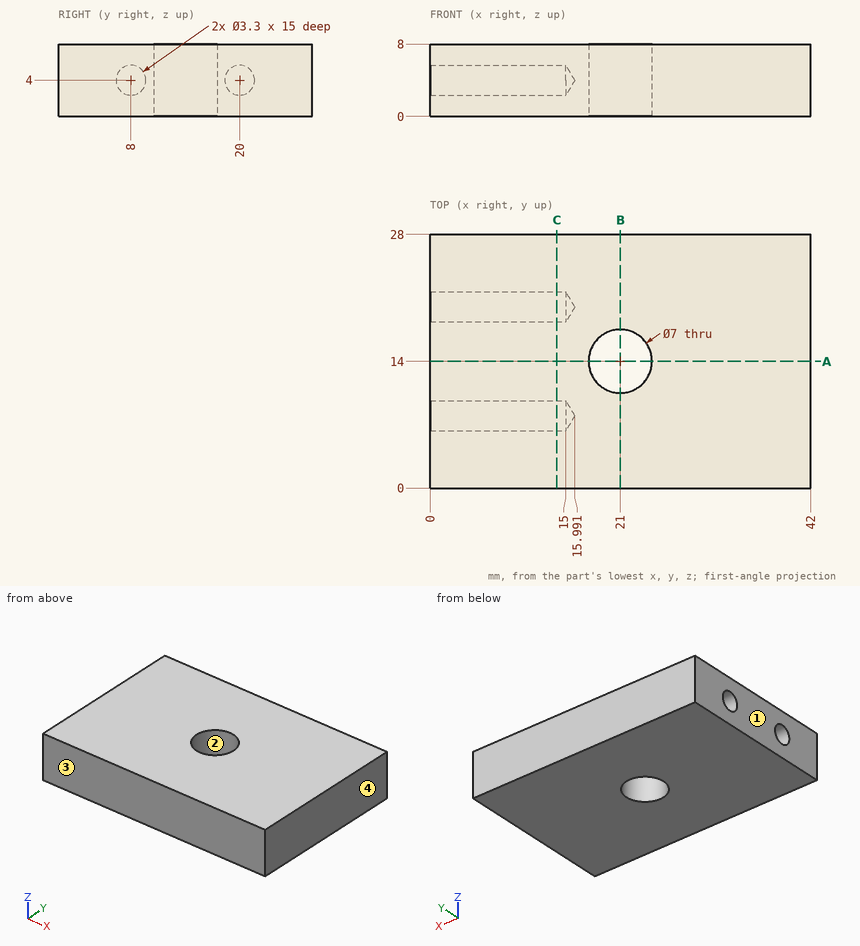
Could you check a few things on this drawing? It's one solid part, dimensions in mm from its lowest x, y, z. Round coordinates to 2 decimals unless told otherwise and drop trailing zeros. Order: outer loops, then holes, each group sorted by start corner. A loop starts at its lowest first (then second) coordinate and runs counter-clockwise, first axis right, second up. Notation, with made-up numbers: M 59.5,-40 L 116.5,-40 A26 cw 116.5,-21 Z; hole C 70.25,33.5 d5. An arc over 180 degrees is marked long. Use a Markdown table: item, result.
1) Imagine slicing it at C-C (x = 14). List the corners of the cut face in (y, z) for me, then the cut area to 3 significant figures.
Geometry says:
| item | result |
|---|---|
| outline | M 0,0 L 28,0 L 28,8 L 0,8 Z; hole C 8,4 d3.3; hole C 20,4 d3.3 |
| area | 207 mm² |
2) If we mould it in two halves opening along X, with no side actions, what happens to the marked faces 1, 2, 3 and 4? For each: +X half, -X half, draft (parallel to the pull), parting line (faces both ways), or undercut.
Geometry says:
| item | result |
|---|---|
| face 1 | -X half |
| face 2 | undercut |
| face 3 | draft |
| face 4 | +X half |
3) I'm going to push a flat-ended pin straight in: P1, Ø3, axis at x = 5.5, y = 22, coming from the -Z side. Where does the tip first touch, or does it pass through?
Geometry says:
| item | result |
|---|---|
| P1 | stops at z = 0 |
4) Imagine slicing it at B-B (x = 21). List the corners of the cut face in (y, z) for me, then the cut area to 3 significant figures.
Geometry says:
| item | result |
|---|---|
| outline | M 0,0 L 10.5,0 L 10.5,8 L 0,8 Z; M 17.5,0 L 28,0 L 28,8 L 17.5,8 Z |
| area | 168 mm² |
5) If I drill on line 1 along Y through (x, z) = (3, 4); line 2 along Z through (x, y) = (7.5, 20); line 3 along X through (y, z) = (13.75, 6), over which ranges is the centre line in solid material (lowest first)?
Geometry says:
| item | result |
|---|---|
| line 1 | y = 0 to 6.35, 9.65 to 18.35, 21.65 to 28 |
| line 2 | z = 0 to 2.35, 5.65 to 8 |
| line 3 | x = 0 to 17.51, 24.49 to 42 |
6) Imagine slicing it at A-A (y = 14). List the corners of the cut face in (x, z) for me.
Geometry says:
| item | result |
|---|---|
| outline | M 0,0 L 17.5,0 L 17.5,8 L 0,8 Z; M 24.5,0 L 42,0 L 42,8 L 24.5,8 Z |
